Job drawing, mm, ordinate dimensions from the low corner. One solid piece. A direction names the side the tool comes from. Give positions to 0.01 mm unless a question says otherwise; leave off trailing zeros. Loops run counter-clockwise (first coordinate to the right, second up) from the corner with the lowest first, then second, coordinate; pieces in that order, holes last.
Item 1: Saw through at D-D on y = 0.6. Give the cut face in (x, z).
Item 2: Which spindle directions (+Z, -Z, +X, -X, +Y, -Y) get a long thin tool onto all of the face, cutting with end or side? Do the marked faces 1, 2 and 3. Say none if no direction does.
Item 3: Saw through at C-C on x = 12.25. Give the cut face in (y, z).
Item 4: Saw through at A-A on z = 3. Give the cut face in (x, y), plus the area to 3 significant figures.
Item 5: Drop flat-ended pins along their axis: P1, Ø1.5, axis at y = 1, z = 1, coming from the +X side; P2, Ø2, axis at x = 10.5, y = 3, coming from the -Z side; P3, Ø2, axis at x = 4.5, y = 2, coming from the -Z side. Give the stop position or say it passes through.
Item 6: Probe probe 1 along X at (y, z) = (1.55, 0.45); probe 2 along Y at (x, z) = (1, 1.9); probe 3 along Z at (x, y) = (8.25, 5.75). List the from-to ranges inside material, lowest first.
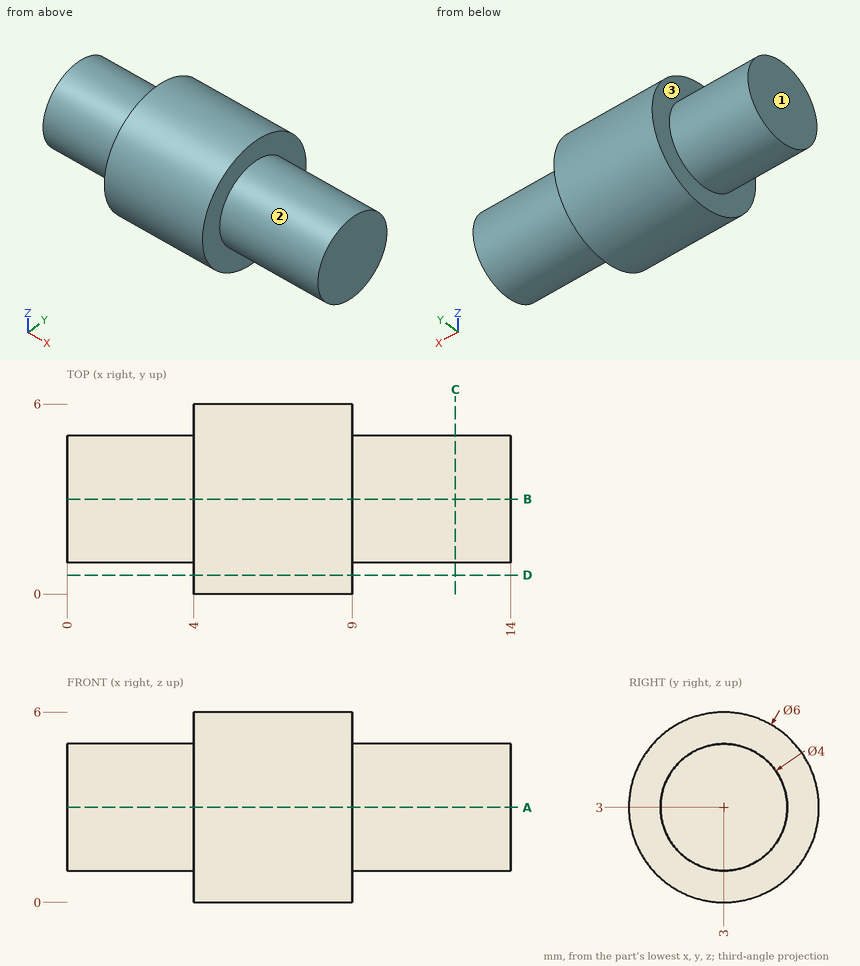
Results below:
1. outline: (4, 1.2) - (9, 1.2) - (9, 4.8) - (4, 4.8) - close
2. face 1: +Z, -Z, -X, +Y, -Y
2. face 2: +X
2. face 3: -X
3. outline: circle Ø4 at (3, 3)
4. outline: (0, 1) - (4, 1) - (4, 0) - (9, 0) - (9, 1) - (14, 1) - (14, 5) - (9, 5) - (9, 6) - (4, 6) - (4, 5) - (0, 5) - close
4. area: 66.0 mm2
5. P1: stops at x = 9
5. P2: stops at z = 1
5. P3: stops at z = 0
6. probe 1: x = 4 to 9
6. probe 2: y = 1.33 to 4.67
6. probe 3: z = 1.8 to 4.2
